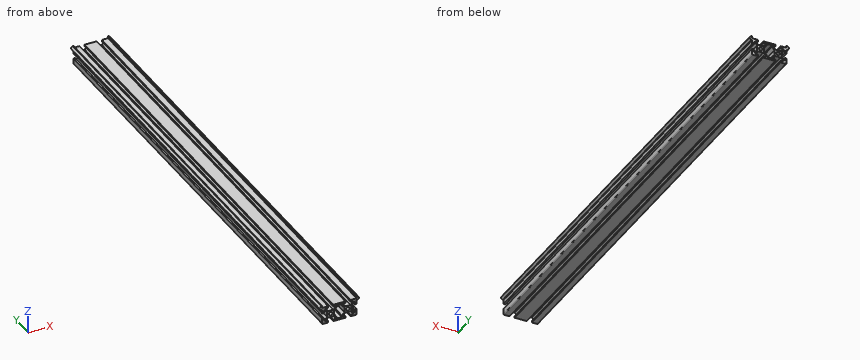
```python
from build123d import *

# Parameters (mm, degrees)
F0_R     = 2.1
F1_DEPTH = 560


with BuildPart() as f1:
    # F0 (on Front) → F1 (new body)
    with BuildSketch(Plane.XZ):
        with BuildLine():
            Line((20, 12.38), (20, 10))
            Line((20, 10), (16, 10))
            Line((16, 10), (13, 10))
            Line((13, 10), (13, 8))
            Line((13, 8), (16, 8))
            Line((16, 8), (16, 7.06))
            Line((16, 7.06), (12.94, 4))
            Line((12.94, 4), (7.06, 4))
            Line((7.06, 4), (4, 7.06))
            Line((4, 7.06), (4, 8))
            Line((4, 8), (2.94, 8))
            Line((2.94, 8), (2.94, 6))
            Line((2.94, 6), (6, 2.94))
            Line((6, 2.94), (6, -2.94))
            Line((6, -2.94), (2.94, -6))
            Line((2.94, -6), (2.94, -8))
            Line((2.94, -8), (4, -8))
            Line((4, -8), (4, -7.06))
            Line((4, -7.06), (7.06, -4))
            Line((7.06, -4), (12.94, -4))
            Line((12.94, -4), (16, -7.06))
            Line((16, -7.06), (16, -8))
            Line((16, -8), (13, -8))
            Line((13, -8), (13, -10))
            Line((13, -10), (16, -10))
            Line((16, -10), (19, -10))
            ThreePointArc((19, -10), (19.707107, -9.707107), (20, -9))
            Line((20, -9), (20, -6))
            Line((20, -6), (20, -3))
            Line((20, -3), (18, -3))
            Line((18, -3), (18, -6))
            Line((18, -6), (17.06, -6))
            Line((17.06, -6), (14, -2.94))
            Line((14, -2.94), (14, 2.94))
            Line((14, 2.94), (17.06, 6))
            Line((17.06, 6), (18, 6))
            Line((18, 6), (18, 3))
            Line((18, 3), (20, 3))
            Line((20, 3), (20, 6))
            Line((20, 6), (20, 7.12))
            ThreePointArc((20, 7.12), (20.146447, 7.473553), (20.5, 7.62))
            Line((20.5, 7.62), (21, 7.62))
            Line((21, 7.62), (23.026447, 9.646447))
            ThreePointArc((23.026447, 9.646447), (23.172893, 10), (23.026447, 10.353553))
            Line((23.026447, 10.353553), (21, 12.38))
            Line((21, 12.38), (20, 12.38))
        make_face()
        with Locations((10, 0)):
            Circle(F0_R, mode=Mode.SUBTRACT)
        Polygon((2.94, 8), (4, 8), (7, 8), (7, 10), (1, 10), (-7, 10), (-7, 8), (-4, 8), (-2.94, 8), align=None)
        with BuildLine():
            Line((-2.94, 6), (-2.94, 8))
            Line((-2.94, 8), (-4, 8))
            Line((-4, 8), (-4, 7.06))
            Line((-4, 7.06), (-7.06, 4))
            Line((-7.06, 4), (-12.94, 4))
            Line((-12.94, 4), (-16, 7.06))
            Line((-16, 7.06), (-16, 8))
            Line((-16, 8), (-13, 8))
            Line((-13, 8), (-13, 10))
            Line((-13, 10), (-16, 10))
            Line((-16, 10), (-20, 10))
            Line((-20, 10), (-20, 12.38))
            Line((-20, 12.38), (-21, 12.38))
            Line((-21, 12.38), (-23.026447, 10.353553))
            ThreePointArc((-23.026447, 10.353553), (-23.172893, 10), (-23.026447, 9.646447))
            Line((-23.026447, 9.646447), (-21, 7.62))
            Line((-21, 7.62), (-20.5, 7.62))
            ThreePointArc((-20.5, 7.62), (-20.146447, 7.473553), (-20, 7.12))
            Line((-20, 7.12), (-20, 6))
            Line((-20, 6), (-20, 3))
            Line((-20, 3), (-18, 3))
            Line((-18, 3), (-18, 6))
            Line((-18, 6), (-17.06, 6))
            Line((-17.06, 6), (-14, 2.94))
            Line((-14, 2.94), (-14, -2.94))
            Line((-14, -2.94), (-17.06, -6))
            Line((-17.06, -6), (-18, -6))
            Line((-18, -6), (-18, -3))
            Line((-18, -3), (-20, -3))
            Line((-20, -3), (-20, -6))
            Line((-20, -6), (-20, -9))
            ThreePointArc((-20, -9), (-19.707107, -9.707107), (-19, -10))
            Line((-19, -10), (-16, -10))
            Line((-16, -10), (-13, -10))
            Line((-13, -10), (-13, -8))
            Line((-13, -8), (-16, -8))
            Line((-16, -8), (-16, -7.06))
            Line((-16, -7.06), (-12.94, -4))
            Line((-12.94, -4), (-7.06, -4))
            Line((-7.06, -4), (-4, -7.06))
            Line((-4, -7.06), (-4, -8))
            Line((-4, -8), (-7, -8))
            Line((-7, -8), (-7, -10))
            Line((-7, -10), (7, -10))
            Line((7, -10), (7, -8))
            Line((7, -8), (4, -8))
            Line((4, -8), (2.94, -8))
            Line((2.94, -8), (-2.94, -8))
            Line((-2.94, -8), (-2.94, -6))
            Line((-2.94, -6), (-6, -2.94))
            Line((-6, -2.94), (-6, 2.94))
            Line((-6, 2.94), (-2.94, 6))
        make_face()
        with Locations((-10, 0)):
            Circle(F0_R, mode=Mode.SUBTRACT)
    extrude(amount=F1_DEPTH)


solid = f1.part
```
For this review, take the finished solid that the model builds, in its own axes (mm). Round coordinates to 2 decimals unless told otherwise and drop trailing zeros. Use a Markdown table: item, result.
Item 1: Take a section at A-A (y = -419). State how many separate pieces and enclosed holes the cut face has, plus the area to 3 significant figures.
Resolved:
| item | result |
|---|---|
| separate pieces | 1 |
| enclosed holes | 3 |
| area | 340 mm² |
Item 2: For line 1 along X through (y, z) = (-330.5, -7.5); line 2 along Z through (x, y) = (10, -351); line 3 along Z through (x, y) = (-19, -403), list the stretches that pass through material, from the lowest coordinate up. Write a range as [from, to].
Resolved:
| item | result |
|---|---|
| line 1 | x = [-20, -16], [-4, -2.94], [2.94, 4], [16, 20] |
| line 2 | z = [-4, -2.1], [2.1, 4] |
| line 3 | z = [-10, -3], [3, 10] |
Item 3: For pin 1 (4 mm diameter, centred on x = -10, z = 0, fed in from +Y); pin 2 (0.5 mm diameter, centred on x = -17.5, y = -210.5, fed in from +Z); pin 3 (10 mm diameter, centred on y = -174, z = 4, fed in from -X); pin 4 (10 mm diameter, centred on y = -322.5, z = -3.5, fed in from +X), all flat-tipped, find the tip position at first contact; note any pin that passes through.
Resolved:
| item | result |
|---|---|
| pin 1 | passes through |
| pin 2 | stops at z = 10 |
| pin 3 | stops at x = -22.38 |
| pin 4 | stops at x = 20 |
